```python
from build123d import *

# Parameters (mm, degrees)
BOSS_EXTRUDE1_DEPTH = 15.85
SHELL1_T            = -1.55
SKETCH2_R           = 1.5
SKETCH2_R_2         = 0.7
BOSS_EXTRUDE2_DEPTH = 1.4
FILLET1_R           = 0.5


with BuildPart() as part:
    # Sketch1 → Boss-Extrude1 (new body)
    with BuildSketch(Plane(origin=(0, 0, 0), x_dir=(0, 0, -1), z_dir=(1, 0, 0))):
        Polygon((0, 0), (7.8, 0), (7.8, 3.15), (1.5, 3.15), (1.5, 9.45), (0, 9.45), align=None)
    extrude(amount=-BOSS_EXTRUDE1_DEPTH)

    # Shell1
    shell1_openings = [part.faces().sort_by_distance(p)[0] for p in [
        (-7.925, 0, -3.9),
    ]]
    offset(amount=SHELL1_T, openings=shell1_openings, kind=Kind.INTERSECTION)

    # Sketch2 → Boss-Extrude2 (add)
    with BuildSketch(Plane.XZ.offset(-1.6)):
        with Locations(Location((-7.925, -3.9, 0), (0, 0, 90))):
            Circle(SKETCH2_R)
        with Locations(Location((-7.925, -3.9, 0), (0, 0, 270))):
            Circle(SKETCH2_R_2, mode=Mode.SUBTRACT)
    extrude(amount=BOSS_EXTRUDE2_DEPTH)

    # Fillet1
    fillet1_edges = [part.edges().sort_by_distance(p)[0] for p in [
        (-15.85, 9.45, -0.75),
        (0, 9.45, -0.75),
    ]]
    fillet(fillet1_edges, radius=FILLET1_R)


solid = part.part
```
Geometry: final body of the model. Coordinates: model frame, mm. A direction names the side the tool comes from. Give positions to 0.01 mm unless a question says otherwise; leave off trailing zeros. Order: outer loops, then holes, each group sorted by start corner. A loop starts at its lowest first (then second) coordinate and runs counter-clockwise, first axis right, second up. Notation, with made-up numbers: (-11.5, -9) -> (-2.5, -9) arc R20 cw to (-2.5, 8) -> close; hole circle Ø8 at (34.5, -22). An arc over 180 degrees is marked (long way). Write each question's results on one line, items separated by ' | '. Start each with the question number.
1) Line query: line 1 (X direction, y = 1.15, z = -3.9) (3 decimals); line 2 (Z direction, x = -9.25, y = 1.5); line 3 (Y direction, x = -11.25, z = -2.75). Output: solid intervals per line, ascending. Write a range as from..to.
2) Draft query along X for faces 4 (the cylindrical face through (-9.41, 0.91, -4.1)), 5 (the flat face through (-8, 6, -1.5)), 6 (the flat face through (0, 2.5, -3)). Return one class per face: pulls with the +X half, pulls with the -X half, needs draft (parallel to the pull), parting line crosses it, or undercut.
3) Section C-C (y = 7.5). Return loops of the section in (x, z).
4) First-contact query: pin 1 (5 mm diameter, centred on x = -6.5, y = 8, fed in from -Z); pin 2 (1.6 mm diameter, centred on x = -7.925, z = -3.9, fed in from +Y); pin 3 (0.9 mm diameter, centred on x = -8, z = -3, fed in from -Y). Flat tips, straight axial feed; report the tip coordinate or a pass-through.
5) Section A-A (x = -3.75). Return loops of the section in (y, z), then the cut area to 3 significant figures.
6) Section D-D (x = -7.75). Return loops of the section in (y, z).
7) Section B-B (z = -3.9). Return loops of the section in (x, y) (3 decimals).
8) Set-up query: faces 1 (the flat face through (-8, 3.15, -5)), 2 (the flat face through (-14.3, 1, -4)), 3 (the flat face through (-8, 2, -7.8)). Return all of +Z, -Z, +X, -X, +Y, -Y with unobstructed straight access to the full face (end or side cutting, diameter ignored); none if empty.
Calculated:
1) line 1: -15.85..-14.3, -9.425..-8.625, -7.225..-6.425, -1.55..0 | line 2: -7.8..-6.25, -4.6..-3.2, -1.55..0 | line 3: 1.6..3.15
2) face 4: undercut | face 5: needs draft | face 6: pulls with the +X half
3) outline: (-15.85, -1.5) -> (0, -1.5) -> (0, 0) -> (-15.85, 0) -> close
4) pin 1: z = -1.5 | pin 2: y = 3.15 | pin 3: y = 0.2
5) outline: (0, -7.8) -> (3.15, -7.8) -> (3.15, -1.5) -> (9.45, -1.5) -> (9.45, 0) -> (0, 0) -> (0, -1.55) -> (1.6, -1.55) -> (1.6, -6.25) -> (0, -6.25) -> close | area: 26.5 mm2
6) outline: (0, -7.8) -> (3.15, -7.8) -> (3.15, -1.5) -> (9.45, -1.5) -> (9.45, 0) -> (0, 0) -> (0, -1.55) -> (1.6, -1.55) -> (1.6, -2.41) -> (0.2, -2.41) -> (0.2, -3.22) -> (1.6, -3.22) -> (1.6, -4.58) -> (0.2, -4.58) -> (0.2, -5.39) -> (1.6, -5.39) -> (1.6, -6.25) -> (0, -6.25) -> close
7) outline: (-15.85, 0) -> (-14.3, 0) -> (-14.3, 1.6) -> (-9.425, 1.6) -> (-9.425, 0.2) -> (-8.625, 0.2) -> (-8.625, 1.6) -> (-7.225, 1.6) -> (-7.225, 0.2) -> (-6.425, 0.2) -> (-6.425, 1.6) -> (-1.55, 1.6) -> (-1.55, 0) -> (0, 0) -> (0, 3.15) -> (-15.85, 3.15) -> close
8) face 1: -Z, +X, -X, +Y | face 2: -Y | face 3: -Z, +X, -X, +Y, -Y
